Part model, mm, in its own coordinate system. A direction names the side the tool comes from. Round coordinates to 2 decimals unless told otherwise and drop trailing zeros. Write each loop counter-clockwise with the first axis right and the second up, starting at its lowest first coordinate (ties: lowest second). Pieces come first, ordered by that corner, then holes. Notation, with made-up numbers: M 19.5,25.25 L 37.5,25.25 A16 cw 37.5,47.25 Z; hole C 85.5,-23 d9. An arc over 180 degrees is marked long. Answer as a JSON object with one key per item and string values. Group by question number.
1. Band-saw the part on A-A, the plane y = 0. Count the separate pieces of the cut face and the enclosed holes in it, plus the area to 3 significant figures.
2. Band-saw the part on B-B, the plane z = 156. Write the cut outline in (x, y), plus the area to 3 significant figures.
3. Band-saw the part on D-D, the plane x = 0. Write the cut outline in (y, z).
4. Band-saw the part on C-C, the plane z = 39. Write the cut outline in (x, y).
5. Two-plate mould, pull along X, no slides. Class faces 1 (the face through (-306.388, 0, -146)), 2 (the face through (7.02, -0.36, 319.01)), 3 (the face through (-352, 0, -292.1)): +X half, -X half, draft (parallel to the pull), parting line (faces both ways), or undercut.
6. Which spindle directions (+Z, -Z, +X, -X, +Y, -Y) get a long thin tool onto all of the face, cutting with end or side? Do faces 4 (the face through (319.088, 0, -145)), 5 (the face through (306.388, 0, -142)), 6 (the face through (-319.088, 0, -141)). Say none if no direction does.
7. Drill centre lines: line 1 (X direction, y = -17, z = -232); line 2 (X direction, y = 0, z = -301.75); line 3 (X direction, y = 0, z = -296.25). Where is each one in solid material? Low to high. Write a range as from..to.
8. Drop flat-ended pins along their axis: pin 1 (11.5 mm diameter, centred on x = -363.54, y = 0, fed in from -Z); pin 2 (10 mm diameter, centred on y = -4, z = 31, fed in from -X); pin 3 (4 mm diameter, centred on y = 2.5, z = -33, fed in from +X); pin 4 (22 mm diameter, centred on x = 363.54, y = 0, fed in from +Z). Give the stop position or say it passes through.
from build123d import *

# Parameters (mm, degrees)
F1_DEPTH = 25.4
F2_R     = 6.35
F3_R     = 15.875
F4_R     = 9.525
F5_DEPTH = 25.4


with BuildPart() as f1:
    # F0 (on Front) → F1 (new body, symmetric)
    with BuildSketch(Plane.XZ):
        with BuildLine():
            Line((306.3875, -304.8), (395.2875, -304.8))
            Line((395.2875, -304.8), (395.2875, -292.1))
            Line((395.2875, -292.1), (319.0875, -292.1))
            Line((319.0875, -292.1), (319.0875, 0))
            ThreePointArc((319.0875, 0), (0, 319.0875), (-319.0875, 0))
            Line((-319.0875, 0), (-319.0875, -292.1))
            Line((-319.0875, -292.1), (-395.2875, -292.1))
            Line((-395.2875, -292.1), (-395.2875, -304.8))
            Line((-395.2875, -304.8), (-306.3875, -304.8))
            Line((-306.3875, -304.8), (-306.3875, 0))
            ThreePointArc((-306.3875, 0), (0, 306.3875), (306.3875, 0))
            Line((306.3875, 0), (306.3875, -304.8))
        make_face()
    extrude(amount=F1_DEPTH, both=True)

    # F2
    f2_edges = [f1.edges().sort_by_distance(p)[0] for p in [
        (-319.0875, 0, -292.1),
        (319.0875, 0, -292.1),
    ]]
    fillet(f2_edges, radius=F2_R)

    # F3
    f3_edges = [f1.edges().sort_by_distance(p)[0] for p in [
        (306.3875, 0, -304.8),
        (-306.3875, 0, -304.8),
    ]]
    fillet(f3_edges, radius=F3_R)

    # F4 (on face) → F5 (cut)
    with BuildSketch(Plane(origin=(0, 0, -304.8), x_dir=(1, 0, 0), z_dir=(0, 0, -1))):
        with Locations((-363.5375, 0)):
            Circle(F4_R)
        with Locations((363.5375, 0)):
            Circle(F4_R)
    extrude(amount=-F5_DEPTH, mode=Mode.SUBTRACT)


solid = f1.part
Worked answers:
{
 "1": {"separate pieces": "3", "enclosed holes": "0", "area": "21,600 mm^2"},
 "2": {"outline": "M -278.35,-25.4 L -263.7,-25.4 L -263.7,25.4 L -278.35,25.4 Z; M 263.7,-25.4 L 278.35,-25.4 L 278.35,25.4 L 263.7,25.4 Z", "area": "1,490 mm^2"},
 "3": {"outline": "M -25.4,306.39 L 25.4,306.39 L 25.4,319.09 L -25.4,319.09 Z"},
 "4": {"outline": "M -316.7,-25.4 L -303.9,-25.4 L -303.9,25.4 L -316.7,25.4 Z; M 303.9,-25.4 L 316.7,-25.4 L 316.7,25.4 L 303.9,25.4 Z"},
 "5": {"face 1": "undercut", "face 2": "parting line", "face 3": "draft"},
 "6": {"face 4": "+Z, +X, +Y, -Y", "face 5": "-Z, +Y, -Y", "face 6": "+Z, -X, +Y, -Y"},
 "7": {"line 1": "x = -319.09..-306.39, 306.39..319.09", "line 2": "x = -395.29..-373.06, -354.01..-312.91, 312.91..354.01, 373.06..395.29", "line 3": "x = -395.29..-373.06, -354.01..-308.18, 308.18..354.01, 373.06..395.29"},
 "8": {"pin 1": "passes through", "pin 2": "stops at x = -318.03", "pin 3": "stops at x = 319.09", "pin 4": "stops at z = -292.1"}
}
